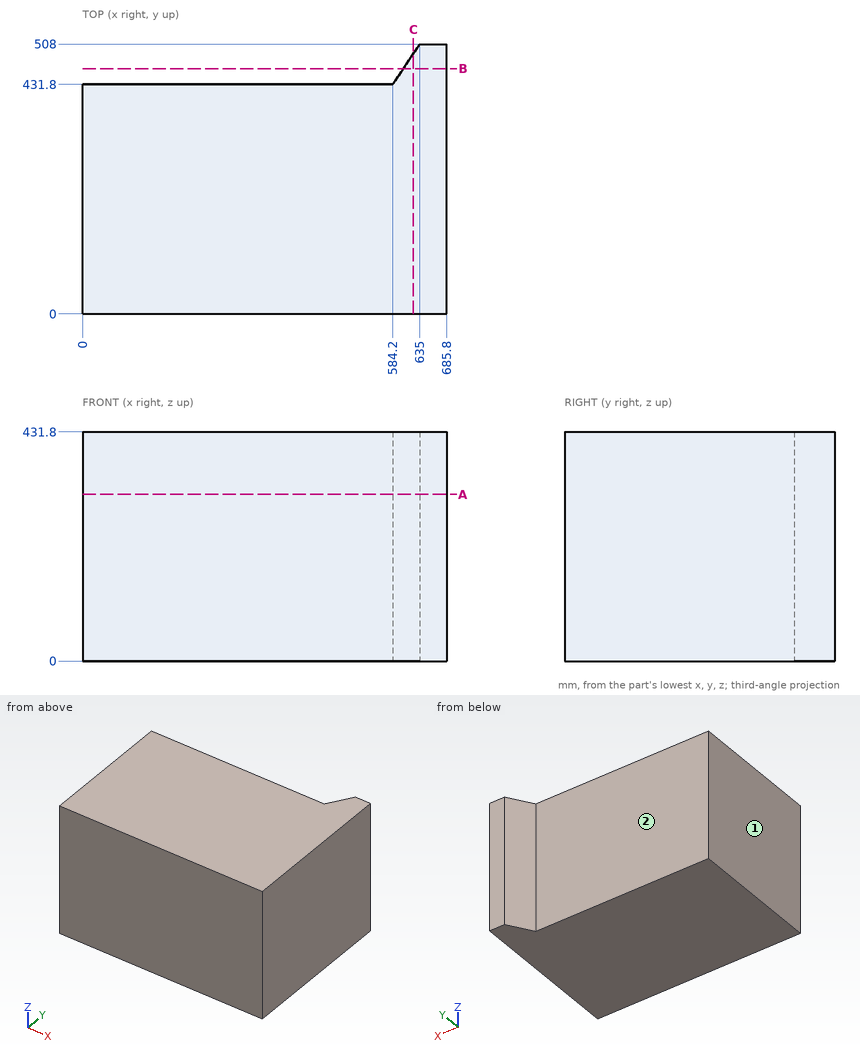
Answer from the drawing. Dimensions are ordinates in mm from the lowest x, y and z of the part. A direction names the side the tool comes from. Coordinates: 2 decimals unless noted, no trailing zeros. Loops run counter-clockwise (first coordinate to the right, second up) from the corner with the lowest first, then second, coordinate; pieces in that order, holes last.
Q1. The part is cut by section B-B on y = 461.5. Write down the section's boundary in (x, z), and give its area (3 significant figures).
Q2. Consider probe 1 along Y at (x, z) = (417, 364); probe 2 along Y at (x, z) = (623, 298); probe 3 along X at (y, z) = (434, 168.5). Determine where each line is inside the solid, lowest interval first.
Q3. Which of the six approach directions +Z, -Z, +X, -X, +Y, -Y give full straight-line access (tool end or side, diameter ignored) to the marked faces 1 and 2?
Q4. This flat-tipped pin is pushed along its axis until it touches: pin 1 Ø10 at (x, z) = (205.5, 76.5) entering from +Y. Where does it stop, or does it pass through?
Q5. The part is cut by section A-A on z = 314. Write down the section's boundary in (x, y).
Q6. The part is cut by section C-C on x = 623. Write down the section's boundary in (y, z).
Results below:
1. outline: (604, 0) - (685.8, 0) - (685.8, 431.8) - (604, 431.8) - close
1. area: 35,300 mm2
2. probe 1: y = 0 to 431.8
2. probe 2: y = 0 to 490
2. probe 3: x = 585.67 to 685.8
3. face 1: +Z, -Z, -X, +Y, -Y
3. face 2: +Z, -Z, -X, +Y
4. pin 1: stops at y = 431.8
5. outline: (0, 0) - (685.8, 0) - (685.8, 508) - (635, 508) - (584.2, 431.8) - (0, 431.8) - close
6. outline: (0, 0) - (490, 0) - (490, 431.8) - (0, 431.8) - close
